Verification items for the finished model (mm, model axes). A direction names the side the tool comes from. Coordinates: 2 decimals unless noted, no trailing zeros. Write each loop counter-clockwise with the first axis right and the second up, starting at its lowest first coordinate (ties: lowest second). Pieces come first, ordered by that corner, then holes. Notation, with made-up numbers: M 77,71 L 121,71 A22 ccw 121,92 Z; hole C 48,50 d6. An arc over 180 degrees is marked long. One line per item, written item: value.
```python
from build123d import *

# Parameters (mm, degrees)
F1_DEPTH = 38.1
F2_R     = 3.175
F3_W     = 19.05
F3_H     = 50.8
F4_DEPTH = 50.801
F5_SIZE  = 5.08


with BuildPart() as f1:
    # F0 (on Front) → F1 (new body)
    with BuildSketch(Plane.XZ):
        with BuildLine():
            Line((9.525, 69.85), (-9.525, 69.85))
            ThreePointArc((-9.525, 69.85), (-20.7503201513, 65.2003201513), (-25.4, 53.975))
            Line((-25.4, 53.975), (-25.4, -53.975))
            ThreePointArc((-25.4, -53.975), (-20.7503201513, -65.2003201513), (-9.525, -69.85))
            Line((-9.525, -69.85), (9.525, -69.85))
            ThreePointArc((9.525, -69.85), (20.7503201513, -65.2003201513), (25.4, -53.975))
            Line((25.4, -53.975), (25.4, 53.975))
            ThreePointArc((25.4, 53.975), (20.7503201513, 65.2003201513), (9.525, 69.85))
        make_face()
    extrude(amount=F1_DEPTH)

    # F2
    f2_edges = [f1.edges().sort_by_distance(p)[0] for p in [
        (25.4, -38.1, 0),
        (25.4, 0, 0),
    ]]
    fillet(f2_edges, radius=F2_R)

    # F3 (on face) → F4 (cut, through all)
    with BuildSketch(Plane.YZ.offset(25.4)):
        with Locations((-19.6936223656, 0)):
            Rectangle(F3_W, F3_H)
    extrude(amount=-F4_DEPTH, mode=Mode.SUBTRACT)

    # F5
    f5_edges = [f1.edges().sort_by_distance(p)[0] for p in [
        (-25.4, -19.05, 53.975),
        (-25.4, -3.175, 0),
        (-25.4, -34.925, 0),
        (-25.4, -19.05, -53.975),
        (-25.4, -19.693622, -25.4),
        (-25.4, -10.168622, 0),
        (-25.4, -19.693622, 25.4),
        (-25.4, -29.218622, 0),
        (25.4, -19.05, -53.975),
        (25.4, -3.175, 0),
        (25.4, -34.925, 0),
        (25.4, -19.05, 53.975),
        (25.4, -29.218622, 0),
        (25.4, -19.693622, 25.4),
        (25.4, -10.168622, 0),
        (25.4, -19.693622, -25.4),
    ]]
    chamfer(f5_edges, length=F5_SIZE)


solid = f1.part
```
Item 1: Scan lines: line 1 (Y direction, x = -18, z = 15); line 2 (Z direction, x = 8, y = -23); line 3 (Z direction, x = -22, y = -13.5). Record each from-to range of solid material in increasing order.
The answers:
line 1: y = -38.1 to -29.22, -10.17 to 0
line 2: z = -69.85 to -25.4, 25.4 to 69.85
line 3: z = -63.79 to -27.08, 27.08 to 63.79
Item 2: Cross-section at C-C, the plane y = -13.5. Enter the section's corners in (x, z) (3 decimals), and give its area (3 significant figures).
The answers:
outline: M -25.4,-53.975 A15.875 ccw -9.525,-69.85 L 9.525,-69.85 A15.875 ccw 25.4,-53.975 L 25.4,-30.48 L 20.32,-25.4 L -20.32,-25.4 L -25.4,-30.48 Z; M -25.4,30.48 L -20.32,25.4 L 20.32,25.4 L 25.4,30.48 L 25.4,53.975 A15.875 ccw 9.525,69.85 L -9.525,69.85 A15.875 ccw -25.4,53.975 Z
area: 4,250 mm²
Item 3: Access from +Z, -Z, +X, -X, +Y, -Y to the whole of each face (thin tool, end or side, straight path). Record for faces 1 (the face through (-22.824, -7.664, -0.427)), 2 (the face through (0, -20, 25.4)), 3 (the face through (22.82, -19.9, 27.9)), 4 (the face through (24.49, -0.95, 0.76)).
The answers:
face 1: -X
face 2: +X, -X
face 3: +X
face 4: +Z, -Z, +X, +Y
Item 4: Draft check along Y on faces 5 (the face through (-25.4, -4.7, 0.8)), 6 (the face through (0, 0, 1)), 7 (the face through (-22.8, -31.7, -0.4)). Enter one of: released by +Y, released by -Y, zero draft, split by the parting line, or undercut.
The answers:
face 5: zero draft
face 6: released by +Y
face 7: undercut
Item 5: Cross-section at D-D, the plane y = -33. Enter the section's corners in (x, z) (3 decimals), and give its area (3 significant figures).
The answers:
outline: M -25.4,-53.975 A15.875 ccw -9.525,-69.85 L 9.525,-69.85 A15.875 ccw 25.4,-53.975 L 25.4,-30.48 L 24.101,-29.181 L 24.101,29.181 L 25.4,30.48 L 25.4,53.975 A15.875 ccw 9.525,69.85 L -9.525,69.85 A15.875 ccw -25.4,53.975 L -25.4,30.48 L -24.101,29.181 L -24.101,-29.181 L -25.4,-30.48 Z
area: 6,730 mm²
Item 6: Cross-section at A-A, the plane z = -3. Enter the section's corners in (x, y) (3 decimals), and give its area (3 significant figures).
The answers:
outline: M -25.4,-34.925 A3.175 ccw -22.225,-38.1 L 22.225,-38.1 A3.175 ccw 25.4,-34.925 L 25.4,-34.299 L 20.32,-29.219 L -20.32,-29.219 L -25.4,-34.299 Z; M -25.4,-5.089 L -20.32,-10.169 L 20.32,-10.169 L 25.4,-5.089 L 25.4,-3.175 A3.175 ccw 22.225,0 L -22.225,0 A3.175 ccw -25.4,-3.175 Z
area: 907 mm²
Item 7: Cross-section at B-B, the plane x = 5.5. Enter the section's corners in (y, z) (3 decimals).
The answers:
outline: M -38.1,-66.675 A3.175 ccw -34.925,-69.85 L -3.175,-69.85 A3.175 ccw 0,-66.675 L 0,66.675 A3.175 ccw -3.175,69.85 L -34.925,69.85 A3.175 ccw -38.1,66.675 Z; hole M -29.219,-25.4 L -10.169,-25.4 L -10.169,25.4 L -29.219,25.4 Z
Item 8: Go/stop test with a flat-tipped pin: P1, Ø5, axis at y = -29.5, z = 9.5, coming from the -X side. Record where the tip stops, or that it passes through.
The answers:
P1: stops at x = -23.1
